Source: CAD feature listing. Evaluate the final solid. Frame: model axes, mm. A direction names the side the tool comes from. Coordinates: 2 decimals unless noted, no trailing zeros. Write each loop counter-clockwise with the first axis right and the second up, starting at its lowest first coordinate (ties: lowest second). Pieces come first, ordered by that corner, then holes. Notation, with made-up numbers: (20.5, -12) -> (33.5, -12) arc R28 cw to (33.5, 24) -> close; hole circle Ø8 at (-5, -17.5). An arc over 180 degrees is marked (long way). Write item = value, one per line.
Autodesk Inventor part; units mm, degrees
ref_plane "Work Plane1" through (0, -7.5, 0) normal (1, 0, 0) x (0, 0, -1)
ref_plane "YZ Plane" through (0, 0, 0) normal (1, 0, 0) x (0, 1, 0)
ref_plane "XZ Plane" through (0, 0, 0) normal (0, 1, 0) x (-1, 0, 0)
sketch "Sketch1" plane through (0, 0, 0) normal (0, 0, 1) x (1, 0, 0)
  line L0 (42.5, -22.5) -> (-42.5, -22.5)
  line L1 (-42.5, -22.5) -> (-42.5, 22.5)
  line L2 (-42.5, 22.5) -> (42.5, 22.5)
  line L3 (42.5, 22.5) -> (42.5, -22.5)
  line L4 (42.5, -22.5) -> (-42.5, 22.5) construction
  line L5 (-42.5, -22.5) -> (42.5, 22.5) construction
  point P0 (0, 0)
  dimension "d0" = 85
  dimension "d1" = 45
extrude "Extrusion1" add sketch "Sketch1" along normal blind 4
sketch "Sketch2" plane through (0, 0, 4) normal (0, 0, 1) x (1, 0, 0)
  line L0 (-42.5, -22.5) -> (42.5, -22.5)
  line L1 (42.5, -22.5) -> (42.5, 22.5)
  line L2 (42.5, 22.5) -> (-42.5, 22.5)
  line L3 (-42.5, 22.5) -> (-42.5, -22.5)
  line L4 (42.5, 17.5) -> (46.5, 17.5)
  line L5 (46.5, 17.5) -> (46.5, 7.5)
  line L6 (46.5, 7.5) -> (42.5, 7.5)
  line L7 (42.5, 7.5) -> (42.5, 17.5)
  line L8 (42.5, -22.5) -> (42.5, 22.5)
  line L9 (42.5, -7.5) -> (46.5, -7.5)
  line L10 (46.5, -7.5) -> (46.5, -17.5)
  line L11 (46.5, -17.5) -> (42.5, -17.5)
  line L12 (42.5, -17.5) -> (42.5, -7.5)
  point P0 (0, 0)
  dimension "d4" = 4
  dimension "d5" = 10
  dimension "d6" = 10
extrude "Extrusion2" add sketch "Sketch2" against normal blind 4 contours L1 L9 L10 L11 | L4 L5 L6 L1
ref_plane "Work Plane1" through (0, -7.5, 0) normal (1, 0, 0) x (0, 0, -1)
mirror "Mirror1" about plane through (0, -7.5, 0) normal (1, 0, 0) of "Extrusion2"
sketch "Sketch3" plane through (0, 0, 4) normal (0, 0, 1) x (1, 0, 0)
  line L0 (-42.5, -22.5) -> (42.5, -22.5)
  line L1 (-32.5, -22.5) -> (-22.5, -22.5)
  line L2 (-22.5, -22.5) -> (-22.5, -30.5)
  line L3 (-22.5, -30.5) -> (-32.5, -30.5)
  line L4 (-32.5, -30.5) -> (-32.5, -22.5)
  line L5 (22.5, -22.5) -> (32.5, -22.5)
  line L6 (32.5, -22.5) -> (32.5, -30.5)
  line L7 (32.5, -30.5) -> (22.5, -30.5)
  line L8 (22.5, -30.5) -> (22.5, -22.5)
  line L9 (-42.5, -17.5) -> (-42.5, -22.5)
  line L10 (42.5, -22.5) -> (42.5, -17.5)
  point P0 (0, 0)
  dimension "d11" = 10
  dimension "d12" = 8
  dimension "d13" = 10
  dimension "d14" = 8
extrude "Extrusion3" add sketch "Sketch3" against normal blind 4
sketch "Sketch4" plane through (0, 0, 4) normal (0, 0, 1) x (1, 0, 0)
  line L0 (42.5, 22.5) -> (-42.5, 22.5)
  line L1 (-32.5, 22.5) -> (-22.5, 22.5)
  line L2 (-22.5, 22.5) -> (-22.5, 26.5)
  line L3 (-22.5, 26.5) -> (-32.5, 26.5)
  line L4 (-32.5, 26.5) -> (-32.5, 22.5)
  line L5 (22.5, 22.5) -> (32.5, 22.5)
  line L6 (32.5, 22.5) -> (32.5, 26.5)
  line L7 (32.5, 26.5) -> (22.5, 26.5)
  line L8 (22.5, 26.5) -> (22.5, 22.5)
  line L9 (-42.5, 22.5) -> (-42.5, 17.5)
  line L10 (42.5, 17.5) -> (42.5, 22.5)
  point P0 (0, 0)
  dimension "d20" = 10
  dimension "d21" = 4
  dimension "d22" = 10
  dimension "d23" = 4
extrude "Extrusion4" add sketch "Sketch4" against normal blind 4
equation "\"d5\" = D"
equation "\"d6\" = D"
equation "\"d11\" = D"
equation "\"d13\" = D"
equation "\"d20\" = D"
equation "\"d22\" = D"
equation "\"D\" = 10"
properties part number "FUENTE 3"
1) Reachability of faces 5 (the flat face through (-42.5, 0, 2)), 6 (the flat face through (-37, -22.5, 2)), 7 (the flat face through (45, 7.5, 2)), 8 (the flat face through (45, -17.5, 2)) from +Z, -Z, +X, -X, +Y, -Y: full face, straight path, thin tool, end or side. Return the list, or none.
Answer block:
face_5 = +Z, -Z, -X
face_6 = +Z, -Z, -X, -Y
face_7 = +Z, -Z, +X
face_8 = +Z, -Z, +X, -Y
2) Cut plane C-C, the plane y = -2.5. Output: boundary loops of the cut face in (x, z).
Answer block:
outline = (-42.5, 0) -> (42.5, 0) -> (42.5, 4) -> (-42.5, 4) -> close
3) Cut plane A-A, the plane y = -24. Output: boundary loops of the cut face in (x, z), and give its area (3 significant figures).
Answer block:
outline = (-32.5, 0) -> (-22.5, 0) -> (-22.5, 4) -> (-32.5, 4) -> close; (22.5, 0) -> (32.5, 0) -> (32.5, 4) -> (22.5, 4) -> close
area = 80.0 mm2
4) Material intervals for probe 1 along X at (y, z) = (-25.5, 1.9); probe 2 along Y at (x, z) = (-1.5, 1.5); probe 3 along X at (y, z) = (4, 3.75), sorted ascending. Write a range as [from, to].
Answer block:
probe_1 = [-32.5, -22.5], [22.5, 32.5]
probe_2 = [-22.5, 22.5]
probe_3 = [-42.5, 42.5]
5) First-contact query: pin 1 Ø2 at (y, z) = (24, 3) entering from +X; pin 2 Ø1.5 at (x, z) = (-3.5, 2.5) entering from -Y; pin 3 Ø1.2 at (x, z) = (-45, 2.5) entering from +Y. Flat tips, straight axial feed; report the tip coordinate or a pass-through.
Answer block:
pin_1 = 32.5
pin_2 = -22.5
pin_3 = 17.5
6) Pull-direction query (X, two-part tool) for faces 1 (the flat face through (0, 22.5, 2)), 2 (the flat face through (-22.5, -26, 2)), 3 (the flat face through (37, 22.5, 2)), 4 (the flat face through (-32.5, -27, 2)); classes: +X half, -X half, draft (parallel to the pull), parting line (faces both ways), or undercut.
Answer block:
face_1 = undercut
face_2 = undercut
face_3 = draft
face_4 = -X half
7) Cut plane B-B, the plane x = 13. Output: boundary loops of the cut face in (y, z), and give its area (3 significant figures).
Answer block:
outline = (-22.5, 0) -> (22.5, 0) -> (22.5, 4) -> (-22.5, 4) -> close
area = 180 mm2
